The figure shows three views and two pictorial views of one solid part (mm, origin at its lowest corner). Answer the questions. A direction names the side the tool comes from. Give positions to 0.01 mm unless a question says otherwise; leave off trailing zeros. Loops run counter-clockwise (first coordinate to the right, second up) from the corner with the lowest first, then second, coordinate; pieces in that order, holes last. Notation, with made-up numbers: M 32,43 L 36,43 A27 cw 36,70 Z; hole C 70,84.25 d3. An arc over 180 degrees is marked long. Write item = value, one per line. Start each with the question number.
1. For the marked faces 1, 2 and 3, determine the directions among +Z, -Z, +X, -X, +Y, -Y from which every point of the face is accessible in a straight line to the end or side of a thin tool.
2. Consider L1, parallel to X at y = 31.5, z = 13.75; L2, parallel to Y at x = 27, z = 11; L3, parallel to X at y = 53.5, z = 5.25. Determine where each line is inside the solid, lowest interval first. Write a range as [from, to].
3. Section B-B on y = 48.1 is taken. Determine the outline of the cut face in (x, z), plus the area to 3 significant figures.
4. Section C-C on x = 5 is taken. Determine the outline of the cut face in (y, z), plus the area to 3 significant figures.
5. Flat-ended cylindrical pins translate along their axes: pin 1 Ø8 at (x, z) = (18, 18) entering from -Y; pin 2 Ø11.5 at (y, z) = (19, 13.5) entering from -X; pin 3 Ø16 at (x, y) = (38, 19.5) entering from -Z. Find the tip coordinate at first contact, or state that the pin passes through.
6. The mould has two halves that part along X. Classify the marked faces 4, 5, 6 and 7: released by +X, released by -X, zero draft, split by the parting line, or undercut.
7. Section D-D on z = 10.5 is taken. Determine the outline of the cut face in (x, y), plus the area to 3 significant figures.
8. Section A-A on z = 2 is taken. Determine the outline of the cut face in (x, y), plus the area to 3 significant figures.
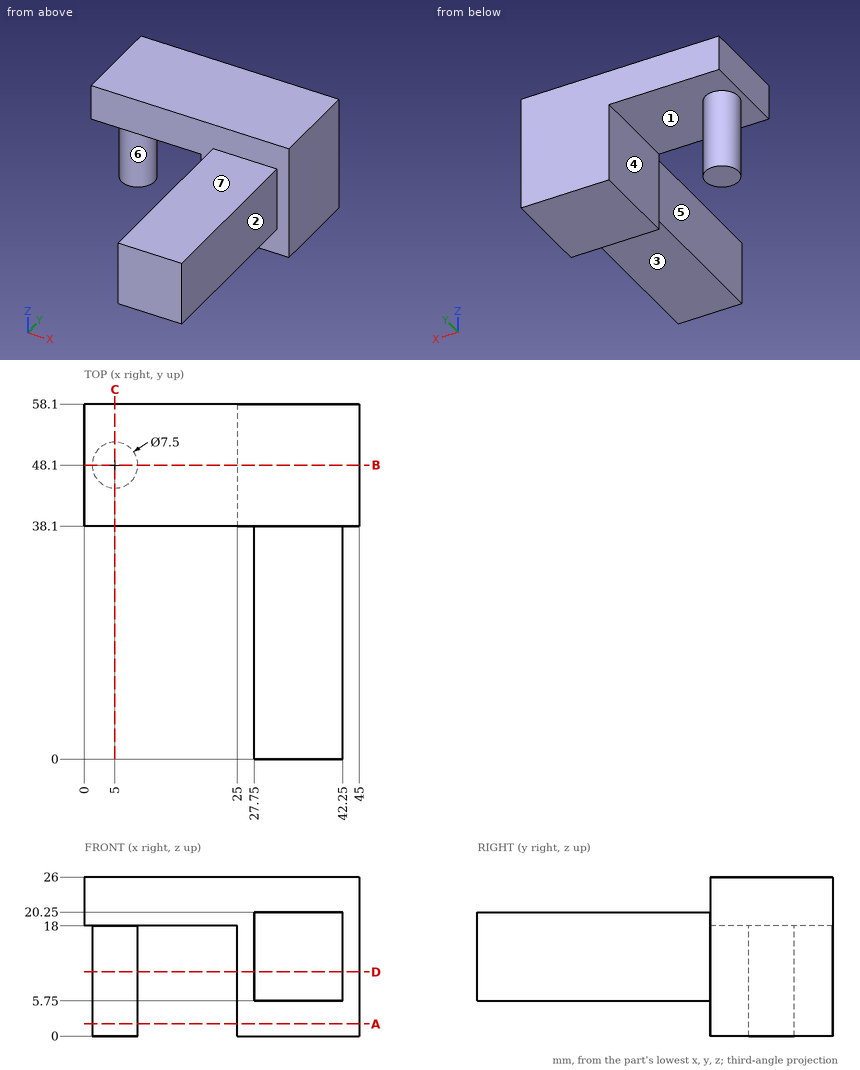
Verdict:
q1.face_1 = -Z
q1.face_2 = +Z, -Z, +X, -Y
q1.face_3 = -Z, +X, -X, -Y
q2.L1 = [27.75, 42.25]
q2.L2 = [38.1, 58.1]
q2.L3 = [25, 45]
q3.outline = M 0,18 L 1.25,18 L 1.25,0 L 8.75,0 L 8.75,18 L 25,18 L 25,0 L 45,0 L 45,26 L 0,26 Z
q3.area = 855 mm2
q4.outline = M 38.1,18 L 44.35,18 L 44.35,0 L 51.85,0 L 51.85,18 L 58.1,18 L 58.1,26 L 38.1,26 Z
q4.area = 295 mm2
q5.pin_1 = 38.1
q5.pin_2 = 27.75
q5.pin_3 = 5.75
q6.face_4 = undercut
q6.face_5 = released by -X
q6.face_6 = undercut
q6.face_7 = zero draft
q7.outline = C 5,48.1 d7.5; M 25,38.1 L 27.75,38.1 L 27.75,0 L 42.25,0 L 42.25,38.1 L 45,38.1 L 45,58.1 L 25,58.1 Z
q7.area = 997 mm2
q8.outline = C 5,48.1 d7.5; M 25,38.1 L 45,38.1 L 45,58.1 L 25,58.1 Z
q8.area = 444 mm2
